Input: part model. Units: mm. Frame: model coordinates. A direction names the side the tool comes from. Round coordinates to 2 decimals unless told otherwise and drop trailing zeros. Loops run counter-clockwise (first coordinate to the right, second up) from the corner with the lowest first, then second, coordinate; pieces in that order, holes last.
(1) Cut plane B-B, the plane z = 0. Output: boundary loops of the cut face in (x, y).
(2) Access query for faces 4 (the face through (-4, 6.9, 4)), 5 (the face through (-3.905, 3.451, -0.867)). Directions: +Z, -Z, +X, -X, +Y, -Y. A direction counts if a zero-diameter tool reaches every point of the face in a straight line with its end or side. Return the directions, or none.
(3) Line query: line 1 (X direction, y = 5.5, z = 0); line 2 (Z direction, x = -1.25, y = 1.5); line 3 (Y direction, x = 8.5, z = -0.5). Output: solid intervals per line, ascending.
(4) Draft query along Z for faces 1 (the face through (-4, 0.1, 4)), 2 (the face through (-10.74, 3.45, -2.38)), 3 (the face through (-2, 7, -4)). Return one class per face: released by +Z, released by -Z, zero draft, split by the parting line, or undercut.
(5) First-contact query: pin 1 Ø9 at (x, z) = (0, 0) entering from +Y; pin 2 Ø1 at (x, y) = (9, 4.5) entering from +Z; pin 3 Ø4 at (x, y) = (-5, 4) entering from +Z. Flat tips, straight axial feed; report the tip coordinate or a pass-through.
(6) Cut plane A-A, the plane x = 0. Output: boundary loops of the cut face in (y, z), and give its area (3 significant figures).
(7) Cut plane C-C, the plane y = 6. Output: boundary loops of the cut face in (x, z).
from build123d import *

# Parameters (mm, degrees)
SKETCH1_R           = 11
SKETCH1_R_2         = 4
BOSS_EXTRUDE1_DEPTH = 7
SKETCH2_R           = 10
SKETCH2_R_2         = 5.5
CUT_EXTRUDE1_DEPTH  = 0.1
FILLET1_R           = 0.25


with BuildPart() as part:
    # Sketch1 → Boss-Extrude1 (new body)
    with BuildSketch(Plane(origin=(0, 0, 0), x_dir=(1, 0, 0), z_dir=(0, 1, 0))):
        with Locations(Location((0, 0, 0), (0, 0, 270))):
            Circle(SKETCH1_R)
        with Locations(Location((0, 0, 0), (0, 0, 270))):
            Circle(SKETCH1_R_2, mode=Mode.SUBTRACT)
    extrude(amount=BOSS_EXTRUDE1_DEPTH)

    # Sketch2 → Cut-Extrude1 (cut)
    with BuildSketch(Plane(origin=(0, 7, 0), x_dir=(1, 0, 0), z_dir=(0, 1, 0))):
        with Locations(Location((0, 0, 0), (0, 0, 270))):
            Circle(SKETCH2_R)
        with Locations(Location((0, 0, 0), (0, 0, 270))):
            Circle(SKETCH2_R_2, mode=Mode.SUBTRACT)
    cut_extrude1 = extrude(amount=-CUT_EXTRUDE1_DEPTH, mode=Mode.SUBTRACT)

    # Mirror1: Cut-Extrude1 across plane
    add(cut_extrude1.mirror(Plane.ZX.offset(3.5)), mode=Mode.SUBTRACT)

    # Fillet1
    fillet1_edges = [part.edges().sort_by_distance(p)[0] for p in [
        (0, 0, -11),
        (0, 7, -11),
    ]]
    fillet(fillet1_edges, radius=FILLET1_R)


solid = part.part
Reported:
1. outline: (-11, 0.25) arc R0.25 ccw to (-10.75, 0) - (-10, 0) - (-10, 0.1) - (-5.5, 0.1) - (-5.5, 0) - (-4, 0) - (-4, 7) - (-5.5, 7) - (-5.5, 6.9) - (-10, 6.9) - (-10, 7) - (-10.75, 7) arc R0.25 ccw to (-11, 6.75) - close; (4, 0) - (5.5, 0) - (5.5, 0.1) - (10, 0.1) - (10, 0) - (10.75, 0) arc R0.25 ccw to (11, 0.25) - (11, 6.75) arc R0.25 ccw to (10.75, 7) - (10, 7) - (10, 6.9) - (5.5, 6.9) - (5.5, 7) - (4, 7) - close
2. face 4: +Y
2. face 5: +Y, -Y
3. line 1: x = -11 to -4, 4 to 11
3. line 2: z = -10.93 to -3.8, 3.8 to 10.93
3. line 3: y = 0.1 to 6.9
4. face 1: undercut
4. face 2: split by the parting line
4. face 3: zero draft
5. pin 1: stops at y = 7
5. pin 2: stops at z = 6.98
5. pin 3: stops at z = 10.58
6. outline: (0, -10.75) arc R0.25 ccw to (0.25, -11) - (6.75, -11) arc R0.25 ccw to (7, -10.75) - (7, -10) - (6.9, -10) - (6.9, -5.5) - (7, -5.5) - (7, -4) - (0, -4) - (0, -5.5) - (0.1, -5.5) - (0.1, -10) - (0, -10) - close; (0, 4) - (7, 4) - (7, 5.5) - (6.9, 5.5) - (6.9, 10) - (7, 10) - (7, 10.75) arc R0.25 ccw to (6.75, 11) - (0.25, 11) arc R0.25 ccw to (0, 10.75) - (0, 10) - (0.1, 10) - (0.1, 5.5) - (0, 5.5) - close
6. area: 96.1 mm2
7. outline: circle Ø22 at (0, 0); hole circle Ø8 at (0, 0)
